from build123d import *

# Parameters (mm, degrees)
F0_W     = 152.4
F0_H     = 80.1413774056
F0_R     = 20.32
F1_DEPTH = 76.2
F2_W     = 66.04
F2_H     = 68.58
F4_DEPTH = 203.2
F5_DEPTH = 203.2
F6_W     = 77.2189535201
F6_H     = 20.4676762223
F7_DEPTH = 25.4


# Not quite as in the source:
# - the program builds the solid bodies; features that only make, move or delete a surface that nothing else refers to are left out


with BuildPart() as f1:
    # F0 (on Front) → F1 (new body)
    with BuildSketch(Plane.XZ):
        with Locations((2.0212908328, 1.0466417298)):
            Rectangle(F0_W, F0_H)
        with Locations((-36.0787091672, 0)):
            Circle(F0_R, mode=Mode.SUBTRACT)
        with Locations((40.1212908328, 0)):
            Circle(F0_R, mode=Mode.SUBTRACT)
    extrude(amount=F1_DEPTH)

    # F2 (on Right) → F4 (cut)
    with BuildSketch(Plane.YZ):
        with Locations((-38.2246004883, 0.5660843734)):
            Rectangle(F2_W, F2_H)
    extrude(amount=-F4_DEPTH, mode=Mode.SUBTRACT)

    # F5 (cut): a face of the model
    f5_faces = [f1.faces().sort_by_distance(p)[0] for p in [
        (0, -38.2246004883, 0.5660843734),
    ]]
    extrude(f5_faces, amount=-F5_DEPTH, mode=Mode.SUBTRACT)

    # F6 (on Top) → F7 (cut)
    with BuildSketch(Plane.XY):
        with Locations((2.0572859794, -37.5628359616)):
            Rectangle(F6_W, F6_H)
    extrude(amount=-F7_DEPTH, mode=Mode.SUBTRACT)


solid = f1.part
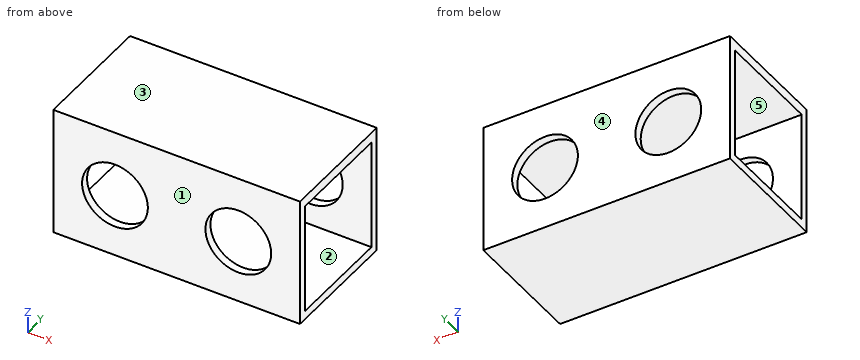
Part model, mm, in its own coordinate system. Face numbers are marked on the shaded views. A direction names the side the tool comes from. Coordinates: 2 decimals unless noted, no trailing zeros. Loops run counter-clockwise (first coordinate to the right, second up) from the corner with the lowest first, then second, coordinate; pieces in that order, holes last. Notation, with made-up numbers: (-4.5, 85.25) -> (41.5, 85.25) arc R22 ccw to (41.5, 115.25) -> close; hole circle Ø9 at (22.25, 16.5). An arc over 180 degrees is marked (long way). Use a Markdown table: item, result. Add a question column.
Item 1: Pull direction Z, two halves, no side cores. Call the marked faces 3, 4 and 5: +Z half, -Z half, draft (parallel to the pull), parting line (faces both ways), or undercut.
Item 2: Which spindle directions (+Z, -Z, +X, -X, +Y, -Y) get a long thin tool onto all of the face, cutting with end or side? Do the marked faces 1 and 2. Say none if no direction does.
Item 3: Probe probe 1 along X at (y, z) = (-2, 0); probe 2 along Y at (x, z) = (-54.5, 34.5); probe 3 along Z at (x, y) = (-18, -21). List the from-to ranges inside material, lowest first.
Item 4: Band-saw the part on A-A on z = 30. Write the cut outline in (x, y).
Item 5: Band-saw the part on D-D on x = -38. Write the cut outline in (y, z).
Item 6: Band-saw the part on C-C on y = -22.5. Write the cut outline in (x, z), plus the area to 3 significant figures.
Item 7: Band-saw the part on B-B on z = 0. Write the cut outline in (x, y), plus the area to 3 significant figures.
Item 8: Flat gauge pins, fed straight in: P1, Ø24.5, axis at x = 40.12, z = 0, coming from the -Y side; P2, Ø20.5, axis at x = -3.5, z = -2.5, coming from the +Y side. Where does each tip first touch, or does it go through?
Geometry says:
| question | item | result |
|---|---|---|
| 1 | face 3 | +Z half |
| 1 | face 4 | draft |
| 1 | face 5 | undercut |
| 2 | face 1 | +Z, -Z, +X, -X, -Y |
| 2 | face 2 | +X, -X |
| 3 | probe 1 | -74.18 to -56.4, -15.76 to 19.8, 60.44 to 78.22 |
| 3 | probe 2 | -76.2 to -71.24, -5.2 to 0 |
| 3 | probe 3 | -39.02 to -33.72, 34.86 to 41.12 |
| 4 | outline | (-74.18, -76.2) -> (78.22, -76.2) -> (78.22, -71.24) -> (-74.18, -71.24) -> close; (-74.18, -5.2) -> (78.22, -5.2) -> (78.22, 0) -> (-74.18, 0) -> close |
| 5 | outline | (-76.2, -39.02) -> (0, -39.02) -> (0, -20.23) -> (-5.2, -20.23) -> (-5.2, -33.72) -> (-71.24, -33.72) -> (-71.24, -20.23) -> (-76.2, -20.23) -> close; (-76.2, 20.23) -> (-71.24, 20.23) -> (-71.24, 34.86) -> (-5.2, 34.86) -> (-5.2, 20.23) -> (0, 20.23) -> (0, 41.12) -> (-76.2, 41.12) -> close |
| 6 | outline | (-74.18, -39.02) -> (78.22, -39.02) -> (78.22, -33.72) -> (-74.18, -33.72) -> close; (-74.18, 34.86) -> (78.22, 34.86) -> (78.22, 41.12) -> (-74.18, 41.12) -> close |
| 6 | area | 1,760 mm² |
| 7 | outline | (-74.18, -76.2) -> (-56.4, -76.2) -> (-56.4, -71.24) -> (-74.18, -71.24) -> close; (-74.18, -5.2) -> (-56.4, -5.2) -> (-56.4, 0) -> (-74.18, 0) -> close; (-15.76, -76.2) -> (19.8, -76.2) -> (19.8, -71.24) -> (-15.76, -71.24) -> close; (-15.76, -5.2) -> (19.8, -5.2) -> (19.8, 0) -> (-15.76, 0) -> close; (60.44, -76.2) -> (78.22, -76.2) -> (78.22, -71.24) -> (60.44, -71.24) -> close; (60.44, -5.2) -> (78.22, -5.2) -> (78.22, 0) -> (60.44, 0) -> close |
| 7 | area | 723 mm² |
| 8 | P1 | through |
| 8 | P2 | y = 0 |
